For this review, take the finished solid that the model builds, in its own axes (mm). Face numbers are marked on the shaded views. A direction names the side the tool comes from. Give positions to 0.01 mm unless a question says otherwise; leave off trailing zeros. Write each loop counter-clockwise with the first axis right and the second up, starting at its lowest first coordinate (ties: lowest second). Pieces come first, ordered by that corner, then holes. Notation, with made-up numbers: (29.5, 78.5) -> (42.5, 78.5) arc R13 cw to (42.5, 85.5) -> close; hole circle Ø7 at (62, -27). An arc over 180 degrees is marked (long way). Write item = value, one per line.
```python
from build123d import *

# Parameters (mm, degrees)
F0_W      = 320
F0_H      = 430
F1_DEPTH  = 5
F2_W      = 35
F2_H      = 100
F3_DEPTH  = 5
F4_W      = 35
F4_H      = 100
F5_DEPTH  = 5
F7_DEPTH  = 5
F8_W      = 3
F8_H      = 70
F9_DEPTH  = 60
F10_W     = 3
F10_H     = 70
F11_DEPTH = 60
F12_W     = 5
F12_H     = 50
F13_DEPTH = 60
F14_W     = 5
F14_H     = 50
F15_DEPTH = 60
F16_R     = 10
F17_DEPTH = 120
F18_R     = 10.2640382995
F19_DEPTH = 240
F20_W     = 10
F20_H     = 15
F21_DEPTH = 30
F22_SIZE  = 14.99999
F23_W     = 10
F23_H     = 15
F24_DEPTH = 30
F25_SIZE  = 14.99999
F26_W     = 10
F26_H     = 60
F27_DEPTH = 40
F28_R     = 5
F29_DEPTH = 240
F30_R     = 5
F31_DEPTH = 240
F32_R     = 5
F33_DEPTH = 250
F34_R     = 5
F35_DEPTH = 300
F36_R     = 5
F37_DEPTH = 300
F38_R     = 5
F39_DEPTH = 300
F40_R     = 10
F41_DEPTH = 207.2868810425
F42_R     = 5
F43_DEPTH = 207.2868810425
F44_R     = 5
F45_DEPTH = 207.2868810425
F46_R     = 5
F47_DEPTH = 207.2868810425
F48_R     = 5
F49_DEPTH = 207.2868810425


# Not quite as in the source:
# - a fillet or chamfer is up to 0.001 mm smaller than in the source, because OpenCascade refuses the exact size


with BuildPart() as f1:
    # F0 (on Top) → F1 (new body)
    with BuildSketch(Plane.XY):
        with Locations((-47.2858810425, 185.3322760761)):
            Rectangle(F0_W, F0_H)
    extrude(amount=F1_DEPTH)

    # F2 (on face) → F3 (cut)
    with BuildSketch(Plane.XY.offset(5)):
        with Locations((-159.7858810425, 171.3026314974)):
            Rectangle(F2_W, F2_H)
    extrude(amount=-F3_DEPTH, mode=Mode.SUBTRACT)

    # F4 (on face) → F5 (cut)
    with BuildSketch(Plane(origin=(0, 0, 0), x_dir=(1, 0, 0), z_dir=(0, 0, -1))):
        with Locations((67.7159577608, -172.2117364407)):
            Rectangle(F4_W, F4_H)
    extrude(amount=-F5_DEPTH, mode=Mode.SUBTRACT)

    # F6 (on face) → F7 (cut)
    with BuildSketch(Plane.XY.offset(5)):
        Polygon((68.7382593751, 362.0384633541), (-166.2617406249, 362.0384633541), (-166.2617406249, 277.0384633541), (-65.0134384632, 277.0384633541), (-48.7617406249, 277.0384633541), (68.7382593751, 277.0384633541), align=None)
    extrude(amount=-F7_DEPTH, mode=Mode.SUBTRACT)

    # F8 (on face) → F9 (join)
    with BuildSketch(Plane.XY.offset(5)):
        with Locations((-205.7858810425, 172.665733695)):
            Rectangle(F8_W, F8_H)
    extrude(amount=F9_DEPTH)

    # F10 (on face) → F11 (join)
    with BuildSketch(Plane.XY.offset(5)):
        with Locations((111.2141189575, 176.3021534681)):
            Rectangle(F10_W, F10_H)
    extrude(amount=F11_DEPTH)

    # F12 (on face) → F13 (join)
    with BuildSketch(Plane.XY.offset(5)):
        with Locations((-204.7858810425, 323.5781848431)):
            Rectangle(F12_W, F12_H)
    extrude(amount=F13_DEPTH)

    # F14 (on face) → F15 (join)
    with BuildSketch(Plane.XY.offset(5)):
        with Locations((110.2141189575, 321.7600047588)):
            Rectangle(F14_W, F14_H)
    extrude(amount=F15_DEPTH)

    # F16 (on Right) → F17 (cut)
    with BuildSketch(Plane.YZ):
        with Locations((175.784942263, 45.0581042336)):
            Circle(F16_R)
    extrude(amount=F17_DEPTH, mode=Mode.SUBTRACT)

    # F18 (on Right) → F19 (cut)
    with BuildSketch(Plane.YZ):
        with Locations((176.2254685163, 45.2939495444)):
            Circle(F18_R)
    extrude(amount=-F19_DEPTH, mode=Mode.SUBTRACT)

    # F20 (on face) → F21 (join)
    with BuildSketch(Plane.XY.offset(5)):
        with Locations((107.7141189575, 18.3457679302)):
            Rectangle(F20_W, F20_H)
    extrude(amount=F21_DEPTH)

    # F22 (size 15 in the source; OpenCascade refuses exactly that, so slightly less here)
    f22_edges = [f1.edges().sort_by_distance(p)[0] for p in [
        (107.714119, 10.845768, 35),
    ]]
    chamfer(f22_edges, length=F22_SIZE)

    # F23 (on face) → F24 (join)
    with BuildSketch(Plane.XY.offset(5)):
        with Locations((-201.83388412, 19.7091826051)):
            Rectangle(F23_W, F23_H)
    extrude(amount=F24_DEPTH)

    # F25 (size 15 in the source; OpenCascade refuses exactly that, so slightly less here)
    f25_edges = [f1.edges().sort_by_distance(p)[0] for p in [
        (-201.833884, 12.209183, 35),
    ]]
    chamfer(f25_edges, length=F25_SIZE)

    # F26 (on face) → F27 (join)
    with BuildSketch(Plane.XY.offset(5)):
        with Locations((-198.1973099709, 328.5773980618)):
            Rectangle(F26_W, F26_H)
    extrude(amount=F27_DEPTH)

    # F28 (on Right) → F29 (cut)
    with BuildSketch(Plane.YZ):
        with Locations((310.6648027897, 53.3718466759)):
            Circle(F28_R)
    extrude(amount=F29_DEPTH, mode=Mode.SUBTRACT)

    # F30 (on Right) → F31 (cut)
    with BuildSketch(Plane.YZ):
        with Locations((330.2825987339, 53.3718466759)):
            Circle(F30_R)
    extrude(amount=F31_DEPTH, mode=Mode.SUBTRACT)

    # F32 (on Right) → F33 (cut)
    with BuildSketch(Plane.YZ):
        with Locations((321.0507035255, 33.1770926714)):
            Circle(F32_R)
    extrude(amount=F33_DEPTH, mode=Mode.SUBTRACT)

    # F34 (on Right) → F35 (cut)
    with BuildSketch(Plane.YZ):
        with Locations((310.0878298283, 52.794855088)):
            Circle(F34_R)
    extrude(amount=-F35_DEPTH, mode=Mode.SUBTRACT)

    # F36 (on Right) → F37 (cut)
    with BuildSketch(Plane.YZ):
        with Locations((330.8595716953, 53.3718466759)):
            Circle(F36_R)
    extrude(amount=-F37_DEPTH, mode=Mode.SUBTRACT)

    # F38 (on Right) → F39 (cut)
    with BuildSketch(Plane.YZ):
        with Locations((321.627676487, 33.7540879846)):
            Circle(F38_R)
    extrude(amount=-F39_DEPTH, mode=Mode.SUBTRACT)

    # F40 (on Right) → F41 (cut, through all)
    with BuildSketch(Plane.YZ):
        with Locations((228.0015647411, 27.0902961493)):
            Circle(F40_R)
    extrude(amount=-F41_DEPTH, mode=Mode.SUBTRACT)

    # F42 (on Right) → F43 (cut, through all)
    with BuildSketch(Plane.YZ):
        with Locations((241.425678134, 41.8319888413)):
            Circle(F42_R)
    extrude(amount=-F43_DEPTH, mode=Mode.SUBTRACT)

    # F44 (on Right) → F45 (cut, through all)
    with BuildSketch(Plane.YZ):
        with Locations((240.8486753702, 12.9823405296)):
            Circle(F44_R)
    extrude(amount=-F45_DEPTH, mode=Mode.SUBTRACT)

    # F46 (on Right) → F47 (cut, through all)
    with BuildSketch(Plane.YZ):
        with Locations((213.0800783634, 41.6209772229)):
            Circle(F46_R)
    extrude(amount=-F47_DEPTH, mode=Mode.SUBTRACT)

    # F48 (on Right) → F49 (cut, through all)
    with BuildSketch(Plane.YZ):
        with Locations((211.7366492748, 12.104251422)):
            Circle(F48_R)
    extrude(amount=-F49_DEPTH, mode=Mode.SUBTRACT)


solid = f1.part
```
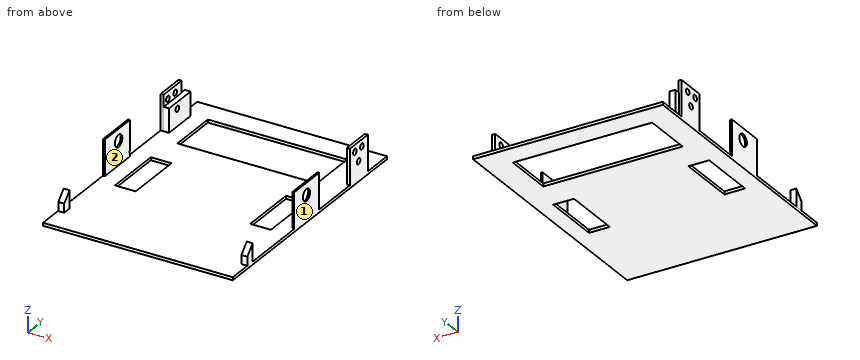
(1) Take a section at D-D (y = 51). Write out the cut boundary in (x, z), plus the area to 3 significant figures.
Answers below:
outline = (-207.29, 0) -> (112.71, 0) -> (112.71, 5) -> (-207.29, 5) -> close
area = 1,600 mm^2
(2) Tool access review of the marked faces 1 and 2: name each direction out of +Z, -Z, +X, -X, +Y, -Y from which nothing blocks a thin tool from reaching the whole face with its end or side.
Answers below:
face_1 = +Z, -Z, +X, +Y, -Y
face_2 = +Z
(3) To check wall thickness, follow probe 1 along X at (y, z) = (150.5, 11.5); probe 2 along Z at (x, y) = (-178, 22.5); probe 3 along Y at (x, z) = (13, 3.5). State the ranges of each line that lie inside material, in increasing order.
Answers below:
probe_1 = -207.29 to -204.29, 109.71 to 112.71
probe_2 = 0 to 5
probe_3 = -29.67 to 277.04, 362.04 to 400.33
(4) Take a section at C-C (x = 21). Write out the cut boundary in (y, z).
Answers below:
outline = (-29.67, 0) -> (277.04, 0) -> (277.04, 5) -> (-29.67, 5) -> close; (362.04, 0) -> (400.33, 0) -> (400.33, 5) -> (362.04, 5) -> close
(5) Take a section at B-B (y = 194.5). Write out the cut boundary in (x, z), plus the area to 3 significant figures.
Answers below:
outline = (-207.29, 0) -> (-177.29, 0) -> (-177.29, 5) -> (-204.29, 5) -> (-204.29, 65) -> (-207.29, 65) -> close; (-142.29, 0) -> (50.22, 0) -> (50.22, 5) -> (-142.29, 5) -> close; (85.22, 0) -> (112.71, 0) -> (112.71, 65) -> (109.71, 65) -> (109.71, 5) -> (85.22, 5) -> close
area = 1,610 mm^2
(6) For pin 1 (2.5 mm diameter, centred on x = -204, z = 46, fed in from -Y); pin 2 (3 mm diameter, centred on x = -198, y = 318, fed in from +Z); pin 3 (11 mm diameter, centred on x = 108, z = 15.5, fed in from -Y); pin 4 (6 mm diameter, centred on y = 321.05, z = 33.18, fed in from +X), all flat-tipped, find the tip position at first contact; note any pin that passes through.
Answers below:
pin_1 = 137.67
pin_2 = 45
pin_3 = 10.85
pin_4 = through
(7) Take a section at A-A (x = -152). Write out the cut boundary in (y, z), plus the area to 4 significant figures.
Answers below:
outline = (-29.67, 0) -> (121.3, 0) -> (121.3, 5) -> (-29.67, 5) -> close; (221.3, 0) -> (277.04, 0) -> (277.04, 5) -> (221.3, 5) -> close; (362.04, 0) -> (400.33, 0) -> (400.33, 5) -> (362.04, 5) -> close
area = 1,225 mm^2
